from build123d import *

# Parameters (mm, degrees)
SKETCH1_W           = 80
SKETCH1_H           = 56
SKETCH1_W_2         = 60.4
SKETCH1_H_2         = 30.2
BOSS_EXTRUDE1_DEPTH = 94
CUT_EXTRUDE1_DEPTH  = 136.543350999
FILLET1_R           = 2


with BuildPart() as part:
    # Sketch1 → Boss-Extrude1 (new body)
    with BuildSketch(Plane.XY):
        with Locations((40, 28)):
            Rectangle(SKETCH1_W, SKETCH1_H)
        with Locations((40, 25.4)):
            Rectangle(SKETCH1_W_2, SKETCH1_H_2, mode=Mode.SUBTRACT)
    extrude(amount=BOSS_EXTRUDE1_DEPTH)

    # Sketch2 → Cut-Extrude1 (cut, through all)
    with BuildSketch(Plane.XY.offset(94)):
        Polygon((9.8, 10.3), (70.2, 10.3), (70.2, 4.2), (74.2, 4.2), (74.2, 0), (70, 0), (10, 0), (5.8, 0), (5.8, 4.2), (9.8, 4.2), align=None)
    extrude(amount=-CUT_EXTRUDE1_DEPTH, mode=Mode.SUBTRACT)

    # Fillet1
    fillet1_edges = [part.edges().sort_by_distance(p)[0] for p in [
        (0, 56, 47),
        (80, 56, 47),
        (80, 0, 47),
        (0, 0, 47),
    ]]
    fillet(fillet1_edges, radius=FILLET1_R)


solid = part.part
Design review of the part built by this model. Coordinates are the model's own, in mm. A direction names the side the tool comes from. Give positions to 0.01 mm unless a question says otherwise; leave off trailing zeros. Write each loop counter-clockwise with the first axis right and the second up, starting at its lowest first coordinate (ties: lowest second). Pieces come first, ordered by that corner, then holes. Notation, with made-up numbers: M 75.5,55.25 L 80.5,55.25 A24 cw 80.5,92.25 Z; hole C 19,0.25 d11. An arc over 180 degrees is marked long. Return JSON: item names as keys, results as strings. Group by question number.
Item 1: Clearance check with flat-ended pins moving along their axes: pin 1 Ø18 at (x, z) = (35.5, 69) entering from -Y; pin 2 Ø12 at (x, y) = (21.5, 8) entering from +Z; pin 3 Ø4.5 at (x, z) = (71, 43) entering from -Y. State where each tip first meets the part, or that it passes through.
Item 2: Take a section at A-A (y = 27.5). Give the boundary of the cut face in (x, z), plus the area to 3 significant figures.
Item 3: The part is to be moulded in two halves that separate along X. For faces 1 (the flat face through (74.2, 2, 48)), 2 (the flat face through (39, 41, 0)), 3 (the flat face through (80, 28, 46)), say which applies: pulls with the +X half, pulls with the -X half, needs draft (parallel to the pull), parting line crosses it, or undercut.
Item 4: Take a section at B-B (z = 86.5). Give the boundary of the cut face in (x, y).
Item 5: Tool access review of faces 4 (the flat face through (0, 28, 46)), 5 (the flat face through (72, 4.2, 48)): name each direction out of +Z, -Z, +X, -X, +Y, -Y from which nothing blocks a thin tool from reaching the whole face with its end or side.
Item 6: Take a section at C-C (x = 42.5). Give the boundary of the cut face in (y, z).
Item 7: Wall thickness on line 1 along X through (y, z) = (22, 72); line 2 along X through (y, z) = (3.5, 55.5); line 3 along Y through (x, z) = (59, 17): over which ranges is each line inside the solid? List them lowest first.
Return value:
{
 "1": {"pin 1": "stops at y = 40.5", "pin 2": "passes through", "pin 3": "stops at y = 4.2"},
 "2": {"outline": "M 0,0 L 9.8,0 L 9.8,94 L 0,94 Z; M 70.2,0 L 80,0 L 80,94 L 70.2,94 Z", "area": "1,840 mm2"},
 "3": {"face 1": "undercut", "face 2": "needs draft", "face 3": "pulls with the +X half"},
 "4": {"outline": "M 0,2 A2 ccw 2,0 L 5.8,0 L 5.8,4.2 L 9.8,4.2 L 9.8,40.5 L 70.2,40.5 L 70.2,4.2 L 74.2,4.2 L 74.2,0 L 78,0 A2 ccw 80,2 L 80,54 A2 ccw 78,56 L 2,56 A2 ccw 0,54 Z"},
 "5": {"face 4": "+Z, -Z, -X, +Y, -Y", "face 5": "+Z, -Z, -Y"},
 "6": {"outline": "M 40.5,0 L 56,0 L 56,94 L 40.5,94 Z"},
 "7": {"line 1": "x = 0 to 9.8, 70.2 to 80", "line 2": "x = 0 to 5.8, 74.2 to 80", "line 3": "y = 40.5 to 56"}
}
